Verification items for the finished model (mm, model axes). Face numbers are marked on the shaded views. A direction names the side the tool comes from. Coordinates: 2 decimals unless noted, no trailing zeros. Order: outer loops, then holes, each group sorted by start corner. A loop starts at its lowest first (then second) coordinate and runs counter-clockwise, first axis right, second up. Notation, with made-up numbers: M 59,38 L 86,38 A6 ccw 86,43 Z; hole C -29.5,-11 d6. An arc over 180 degrees is marked long. Answer as a JSON object with one key per item and string values. Group by question number.
(1) Cross-section at D-D (y = -23). Enter the section's corners in (x, z).
(2) Gauge pin test, flat ends, axial feed: pin 1 Ø2 at (y, z) = (-47.5, 5.5) entering from -X; pin 2 Ø2.5 at (y, z) = (-22, 1.5) entering from -X; pin 3 Ø1.5 at (y, z) = (-31, 2.5) entering from +X; pin 4 Ø6.5 at (x, y) = (10, -49) entering from -Z. Record the tip position at first contact, or that the pin passes through.
(3) Material ranges on line 1 (Z direction, x = 0, y = -45.5) (3 decimals); line 2 (X direction, y = -45, z = 2.75); line 3 (X direction, y = -32.5, z = 0.5), recorded low to high.
(4) Access from +Z, -Z, +X, -X, +Y, -Y to the whole of each face (thin tool, end or side, straight path). Record for the marked faces 1, 2, 3 and 4.
(5) Cross-section at C-C (x = 11.5). Enter the section's corners in (y, z) (3 decimals), plus the area to 4 significant figures.
(6) Cross-section at A-A (y = -45). Enter the section's corners in (x, z) (3 decimals).
(7) Cross-section at B-B (z = 6). Enter the section's corners in (x, y).
(8) Mould release check, pull along Y, two halves, no side actions. Record for the marked faces 5, 6 and 7: released by +Y, released by -Y, zero draft, split by the parting line, or undercut.
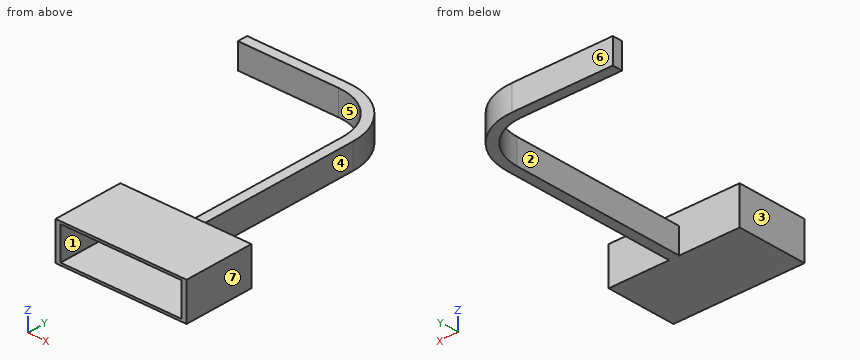
from build123d import *

# Parameters (mm, degrees)
F1_DEPTH = 5
F2_DEPTH = 7.5
F3_W     = 12
F3_H     = 3.275
F4_DEPTH = 13


with BuildPart() as f1:
    # F0 (on Top) → F1 (new body)
    with BuildSketch(Plane.XY):
        with BuildLine():
            Line((-25, 5), (-5, 5))
            Line((-5, 5), (1.6332495807, 5))
            ThreePointArc((1.6332495807, 5), (-1.5358983849, 6.4891252931), (-5, 7))
            Line((-5, 7), (-25, 7))
            Line((-25, 7), (-25, 6))
            Line((-25, 6), (-25, 5))
        make_face()
        with BuildLine():
            Line((1.6332495807, 5), (-5, 5))
            ThreePointArc((-5, 5), (2.0710678119, 2.0710678119), (5, -5))
            Line((5, -5), (5, 1.6332495807))
            ThreePointArc((5, 1.6332495807), (3.4852813742, 3.4852813742), (1.6332495807, 5))
        make_face()
        with BuildLine():
            Line((5, 1.6332495807), (5, -5))
            Line((5, -5), (5, -40))
            Line((5, -40), (6, -40))
            Line((6, -40), (7, -40))
            Line((7, -40), (7, -5))
            ThreePointArc((7, -5), (6.4891252931, -1.5358983849), (5, 1.6332495807))
        make_face()
    extrude(amount=F1_DEPTH)

    # F0 (on Top) → F2 (join)
    with BuildSketch(Plane.XY):
        Polygon((6, -40), (5, -40), (-7, -40), (-7, -54), (6, -54), align=None)
        Polygon((7, -40), (6, -40), (6, -54), (19, -54), (19, -40), align=None)
    extrude(amount=F2_DEPTH)

    # F3 (on face) → F4 (cut)
    with BuildSketch(Plane.XZ.offset(54)):
        with Locations((0, 5.3875)):
            Rectangle(F3_W, F3_H)
        with Locations((12, 5.3875)):
            Rectangle(F3_W, F3_H)
        with Locations((12, 2.1125)):
            Rectangle(F3_W, F3_H)
        with Locations((0, 2.1125)):
            Rectangle(F3_W, F3_H)
    extrude(amount=-F4_DEPTH, mode=Mode.SUBTRACT)


solid = f1.part
Taken from the geometry:
{
 "1": {"outline": "M 5,0 L 7,0 L 7,5 L 5,5 Z"},
 "2": {"pin 1": "stops at x = -7", "pin 2": "stops at x = 5", "pin 3": "stops at x = 7", "pin 4": "stops at z = 0"},
 "3": {"line 1": "z = 0 to 0.475, 7.025 to 7.5", "line 2": "x = -7 to -6, 18 to 19", "line 3": "x = 5 to 7"},
 "4": {"face 1": "-Y", "face 2": "+Z, -Z, -X", "face 3": "+Z, -Z, -X, -Y", "face 4": "+Z, -Z, +X, +Y"},
 "5": {"outline": "M -54,0 L -40,0 L -40,7.5 L -54,7.5 L -54,7.025 L -41,7.025 L -41,0.475 L -54,0.475 Z", "area": "19.85 mm²"},
 "6": {"outline": "M -7,0 L 19,0 L 19,7.5 L -7,7.5 Z; hole M -6,0.475 L 18,0.475 L 18,7.025 L -6,7.025 Z"},
 "7": {"outline": "M -7,-54 L -6,-54 L -6,-41 L 18,-41 L 18,-54 L 19,-54 L 19,-40 L -7,-40 Z"},
 "8": {"face 5": "undercut", "face 6": "released by +Y", "face 7": "zero draft"}
}
